from build123d import *

# Parameters (mm, degrees)
SKETCH1_W           = 65
SKETCH1_H           = 65
SKETCH1_R           = 1.5
BOSS_EXTRUDE1_DEPTH = 6


with BuildPart() as part:
    # Sketch1 → Boss-Extrude1 (new body)
    with BuildSketch(Plane.XY):
        with Locations((19.9, 22.5)):
            Rectangle(SKETCH1_W, SKETCH1_H)
        with Locations((-3.6, 4.65)):
            Circle(SKETCH1_R, mode=Mode.SUBTRACT)
        with Locations((43.4, 4.65)):
            Circle(SKETCH1_R, mode=Mode.SUBTRACT)
        with Locations((-3.6, 24.65)):
            Circle(SKETCH1_R, mode=Mode.SUBTRACT)
        with Locations((43.4, 24.65)):
            Circle(SKETCH1_R, mode=Mode.SUBTRACT)
        with Locations((-3.6, 44.65)):
            Circle(SKETCH1_R, mode=Mode.SUBTRACT)
        with Locations((43.4, 44.65)):
            Circle(SKETCH1_R, mode=Mode.SUBTRACT)
        Polygon((0, 0), (39.8, 0), (39.3, 9.3), (0.5, 9.3), align=None, mode=Mode.SUBTRACT)
    extrude(amount=BOSS_EXTRUDE1_DEPTH)


solid = part.part
For this review, take the finished solid that the model builds, in its own axes (mm). A direction names the side the tool comes from. Round coordinates to 2 decimals unless told otherwise and drop trailing zeros. Loops run counter-clockwise (first coordinate to the right, second up) from the corner with the lowest first, then second, coordinate; pieces in that order, holes last. Notation, with made-up numbers: (-5.5, -24) - (18.5, -24) arc R11 cw to (18.5, -17) - close; hole circle Ø2 at (-28.5, -9). An arc over 180 degrees is marked (long way). One line per question, with ' | ' between items.
Q1. Take a section at B-B (x = 7). Give the boundary of the cut face in (y, z), and give its area (3 significant figures).
Taken from the geometry:
outline: (-10, 0) - (0, 0) - (0, 6) - (-10, 6) - close; (9.3, 0) - (55, 0) - (55, 6) - (9.3, 6) - close | area: 334 mm²
Q2. For line 1 along Y through (x, z) = (43.4, 3.2); line 2 along Y through (x, z) = (17.5, 3.95); line 3 along X through (y, z) = (9, 5.45), list the stretches that pass through material, from the lowest coordinate up. Write a range as [from, to].
Taken from the geometry:
line 1: y = [-10, 3.15], [6.15, 23.15], [26.15, 43.15], [46.15, 55] | line 2: y = [-10, 0], [9.3, 55] | line 3: x = [-12.6, 0.48], [39.32, 52.4]
Q3. Tool access review of faces 1 (the flat face through (20, 0, 3)), 2 (the flat face through (19, 23, 0)): name each direction out of +Z, -Z, +X, -X, +Y, -Y from which nothing blocks a thin tool from reaching the whole face with its end or side.
Taken from the geometry:
face 1: +Z, -Z | face 2: -Z, +X, -X, +Y, -Y
Q4. Take a section at A-A (z = 3.35). Give the boundary of the cut face in (x, y), and give its area (3 significant figures).
Taken from the geometry:
outline: (-12.6, -10) - (52.4, -10) - (52.4, 55) - (-12.6, 55) - close; hole circle Ø3 at (-3.6, 4.65); hole circle Ø3 at (-3.6, 24.65); hole circle Ø3 at (-3.6, 44.65); hole (0, 0) - (39.8, 0) - (39.3, 9.3) - (0.5, 9.3) - close; hole circle Ø3 at (43.4, 4.65); hole circle Ø3 at (43.4, 24.65); hole circle Ø3 at (43.4, 44.65) | area: 3,820 mm²
Q5. Take a section at C-C (y = 4.65). Give the boundary of the cut face in (x, z), and give its area (3 significant figures).
Taken from the geometry:
outline: (-12.6, 0) - (-5.1, 0) - (-5.1, 6) - (-12.6, 6) - close; (-2.1, 0) - (0.25, 0) - (0.25, 6) - (-2.1, 6) - close; (39.55, 0) - (41.9, 0) - (41.9, 6) - (39.55, 6) - close; (44.9, 0) - (52.4, 0) - (52.4, 6) - (44.9, 6) - close | area: 118 mm²
Q6. Take a section at D-D (x = -3.6). Give the boundary of the cut face in (y, z).
Taken from the geometry:
outline: (-10, 0) - (3.15, 0) - (3.15, 6) - (-10, 6) - close; (6.15, 0) - (23.15, 0) - (23.15, 6) - (6.15, 6) - close; (26.15, 0) - (43.15, 0) - (43.15, 6) - (26.15, 6) - close; (46.15, 0) - (55, 0) - (55, 6) - (46.15, 6) - close
Q7. For pin 1 (2.5 mm diameter, centred on x = -3.6, y = 44.65, fed in from +Z), flat-tipped, find the tip position at first contact; note if it passes through.
Taken from the geometry:
pin 1: passes through
